from build123d import *

# Parameters (mm, degrees)
F0_R     = 7
F1_DEPTH = 6
F2_R     = 5.25
F3_DEPTH = 30
F5_DEPTH = 1
F6_R     = 2


with BuildPart() as f1:
    # F0 (on Front) → F1 (new body)
    with BuildSketch(Plane.XZ):
        Circle(F0_R)
    extrude(amount=F1_DEPTH)

    # F2 (on face) → F3 (join)
    with BuildSketch(Plane.XZ.offset(6)):
        Circle(F2_R)
    extrude(amount=F3_DEPTH)

    # F4 (on face) → F5 (cut)
    with BuildSketch(Plane(origin=(0, 0, 0), x_dir=(-1, 0, 0), z_dir=(0, 1, 0))):
        with BuildLine():
            Line((-2.4702025112, 9.5145767555), (-3, 9.5145767555))
            Line((-3, 9.5145767555), (-3, 6.3245553203))
            ThreePointArc((-3, 6.3245553203), (0, 7), (3, 6.3245553203))
            Line((3, 6.3245553203), (3, 9.5145767555))
            Line((3, 9.5145767555), (-2.4702025112, 9.5145767555))
        make_face()
        with BuildLine():
            ThreePointArc((3, -6.3245553203), (0, -7), (-3, -6.3245553203))
            Line((-3, -6.3245553203), (-3, -11.1439647153))
            Line((-3, -11.1439647153), (3, -11.1439647153))
            Line((3, -11.1439647153), (3, -6.3245553203))
        make_face()
        with BuildLine():
            ThreePointArc((3, 6.3245553203), (0, 7), (-3, 6.3245553203))
            Line((-3, 6.3245553203), (-3, -6.3245553203))
            ThreePointArc((-3, -6.3245553203), (0, -7), (3, -6.3245553203))
            Line((3, -6.3245553203), (3, 6.3245553203))
        make_face()
    extrude(amount=-F5_DEPTH, mode=Mode.SUBTRACT)

    # F6
    f6_edges = [f1.edges().sort_by_distance(p)[0] for p in [
        (-5.25, -36, 0),
    ]]
    fillet(f6_edges, radius=F6_R)


solid = f1.part
Can you work these out from the model? Positions are in its coordinate system, mm. A direction names the side the tool comes from. Round coordinates to 2 decimals unless told otherwise and drop trailing zeros. Loops run counter-clockwise (first coordinate to the right, second up) from the corner with the lowest first, then second, coordinate; pieces in that order, holes last. Notation, with made-up numbers: (22, 63) - (40, 63) arc R9 cw to (40, 76) - close; hole circle Ø7 at (73.5, 87.25). An arc over 180 degrees is marked (long way). Answer in a Markdown table with one row per item. Add a question column.
Q1. We'd pull the mould along X, two halves only. Please class faces 4 (the cylindrical face through (5, -19.8, 1.6)), 5 (the flat face through (-3, -0.5, -0.1)), 6 (the flat face through (0, -36, 0)): pulls with the +X half, pulls with the -X half, needs draft (parallel to the pull), parting line crosses it, or undercut.
Q2. I want a section at B-B on z = 0. List the corners of the cut face in (x, y) for me, and give its area (3 significant figures).
Q3. I want a section at A-A on x = 0. List the corners of the cut face in (y, z) for me, and give its area (3 significant figures).
Q4. I need wall thicknesses on L1, parallel to X at y = -4, z = 3; L2, parallel to Z at x = 0.25, y = -28.5; L3, parallel to Y at x = 1.5, z = -2.5. Which ranges of each line are inside material? Lowest first, please.
Q5. Which directions (+Z, -Z, +X, -X, +Y, -Y) give clear straight access to the entire face, cutting with the end or side of a thin tool? Please do faces 1 (the cylindrical face through (6.677, -2.958, 2.103)), 2 (the flat face through (3, -0.5, 0.1)), 3 (the flat face through (3, -6, 5)).
Q6. For pin 1 Ø1.5 at (x, z) = (-2.5, -4.5) entering from +Y; pin 2 Ø0.5 at (y, z) = (-0.5, 2.5) entering from +X; pin 3 Ø3 at (x, y) = (-4.5, -22) entering from +Z; pin 4 Ø1 at (x, y) = (2.5, -21) entering from +Z, each with a flat end and sliding along its axis, tell me the tip position at first contact or that it passes through.
Q7. I want a section at C-C on y = -8. List the corners of the cut face in (x, z) for me.
A:
| question | item | result |
|---|---|---|
| 1 | face 4 | parting line crosses it |
| 1 | face 5 | undercut |
| 1 | face 6 | needs draft |
| 2 | outline | (-7, -6) - (-5.25, -6) - (-5.25, -34) arc R2 ccw to (-3.25, -36) - (3.25, -36) arc R2 ccw to (5.25, -34) - (5.25, -6) - (7, -6) - (7, 0) - (3, 0) - (3, -1) - (-3, -1) - (-3, 0) - (-7, 0) - close |
| 2 | area | 391 mm^2 |
| 3 | outline | (-36, -3.25) arc R2 ccw to (-34, -5.25) - (-6, -5.25) - (-6, -7) - (-1, -7) - (-1, 7) - (-6, 7) - (-6, 5.25) - (-34, 5.25) arc R2 ccw to (-36, 3.25) - close |
| 3 | area | 383 mm^2 |
| 4 | L1 | -6.32 to 6.32 |
| 4 | L2 | -5.24 to 5.24 |
| 4 | L3 | -36 to -1 |
| 5 | face 1 | +Y, -Y |
| 5 | face 2 | +Z, -Z, +Y |
| 5 | face 3 | -Y |
| 6 | pin 1 | y = 0 |
| 6 | pin 2 | x = 6.63 |
| 6 | pin 3 | z = 4.31 |
| 6 | pin 4 | z = 4.85 |
| 7 | outline | circle Ø10.5 at (0, 0) |
